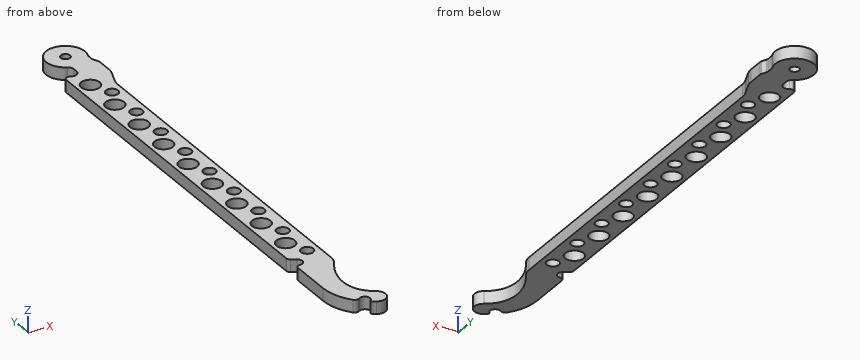
from build123d import *

# Parameters (mm, degrees)
EXTRUDE_1_DEPTH     = 6
CUT_EXTRUDE_1_DEPTH = 7.0000001
HOLE_WIZARD_M41_D   = 4.5
CUT_EXTRUDE_2_DEPTH = 7.0000001
SKETCH_9_R          = 3
SKETCH_9_R_2        = 4.5
CUT_EXTRUDE_4_DEPTH = 7.0000001
CUT_EXTRUDE_6_DEPTH = 7.0000001
FILLET_4_R          = 2
FILLET_5_R          = 10
FILLET_6_R          = 1
FILLET_7_R          = 3


with BuildPart() as part:
    # Эскиз1 → Бобышка-Вытянуть1 (new body)
    with BuildSketch(Plane.XY):
        with BuildLine():
            Line((6.5, -30), (6.5, -210))
            add(Edge.make_bspline(
                [(7.75, -241.602885683), (-4.554007881, -234.499163421), (-0.209884915, -217.844238119), (6.5, -210)],
                knots=[0, 0, 0, 0, 1, 1, 1, 1], degree=3))
            ThreePointArc((7.75, -241.602885683), (9.397114317, -247.75), (3.25, -249.397114317))
            ThreePointArc((3.25, -249.397114317), (1.977735046, -248.713449013), (0.749010369, -247.954310008))
            Line((0.749010369, -247.954310008), (1.25, -247.665063509))
            ThreePointArc((1.25, -247.665063509), (2.165063509, -244.25), (-1.25, -243.334936491))
            Line((-1.25, -243.334936491), (-3.342048726, -244.542781386))
            ThreePointArc((-3.342048726, -244.542781386), (-8.273241088, -236.903089302), (-10, -227.975611669))
            Line((-10, -227.975611669), (-10, 0))
            ThreePointArc((-10, 0), (0, 10), (10, 0))
            Line((10, 0), (10, -20.383829032))
            Line((10, -20.383829032), (6.5, -30))
        make_face()
    extrude(amount=EXTRUDE_1_DEPTH)

    # Эскиз2 → Вырез-Вытянуть1 (cut, through all)
    with BuildSketch(Plane.XY.offset(6)):
        with BuildLine():
            Line((-6.59421021, -201.178331294), (-10, -199.211997642))
            Line((-10, -199.211997642), (-10, -204.985500334))
            Line((-10, -204.985500334), (-9.09421021, -205.508458313))
            ThreePointArc((-9.09421021, -205.508458313), (-5.6791467, -204.593394804), (-6.59421021, -201.178331294))
        make_face()
    extrude(amount=-CUT_EXTRUDE_1_DEPTH, mode=Mode.SUBTRACT)

    # Отверстие с зазором M41 (through all)
    with Locations(Plane.XY.offset(6)):
        with Locations((0, 0)):
            Hole(HOLE_WIZARD_M41_D / 2)

    # Эскиз6 → Вырез-Вытянуть2 (cut, through all)
    with BuildSketch(Plane.XY.offset(6)):
        with BuildLine():
            ThreePointArc((8.758748453, -3.313367558), (-3.216437094, 8.794805936), (-4.554549196, -8.182307784))
            ThreePointArc((-4.554549196, -8.182307784), (-3.004971936, -13.622786652), (-8.445450804, -15.172363912))
            ThreePointArc((-8.445450804, -15.172363912), (-5.964204156, 16.308112544), (16.241251547, -6.143941255))
            ThreePointArc((16.241251547, -6.143941255), (11.084713151, -8.469905953), (8.758748453, -3.313367558))
        make_face()
    extrude(amount=-CUT_EXTRUDE_2_DEPTH, mode=Mode.SUBTRACT)

    # Эскиз9 → Вырез-Вытянуть4 (cut, through all)
    with BuildSketch(Plane.XY.offset(6)):
        with Locations((1, -36.464522083)):
            Circle(SKETCH_9_R)
        with Locations((1, -56.464522083)):
            Circle(SKETCH_9_R)
        with Locations((1, -76.464522083)):
            Circle(SKETCH_9_R)
        with Locations((1, -96.464522083)):
            Circle(SKETCH_9_R)
        with Locations((1, -116.464522083)):
            Circle(SKETCH_9_R)
        with Locations((1, -136.464522083)):
            Circle(SKETCH_9_R)
        with Locations((1, -156.464522083)):
            Circle(SKETCH_9_R)
        with Locations((1, -176.464522083)):
            Circle(SKETCH_9_R)
        with Locations((1, -196.464522083)):
            Circle(SKETCH_9_R)
        with Locations((-3.5, -26.464522083)):
            Circle(SKETCH_9_R_2)
        with Locations((-3.5, -46.464522083)):
            Circle(SKETCH_9_R_2)
        with Locations((-3.5, -66.464522083)):
            Circle(SKETCH_9_R_2)
        with Locations((-3.5, -86.464522083)):
            Circle(SKETCH_9_R_2)
        with Locations((-3.5, -106.464522083)):
            Circle(SKETCH_9_R_2)
        with Locations((-3.5, -126.464522083)):
            Circle(SKETCH_9_R_2)
        with Locations((-3.5, -146.464522083)):
            Circle(SKETCH_9_R_2)
        with Locations((-3.5, -166.464522083)):
            Circle(SKETCH_9_R_2)
        with Locations((-3.5, -186.464522083)):
            Circle(SKETCH_9_R_2)
    extrude(amount=-CUT_EXTRUDE_4_DEPTH, mode=Mode.SUBTRACT)

    # Эскиз11 → Вырез-Вытянуть6 (cut, through all)
    with BuildSketch(Plane.XY.offset(6)):
        Polygon((-2.5, -9.32593934), (-2.5, -18.481802874), (-10, -14.307049262), (-10, -5.151185729), align=None)
        Polygon((10, -7.851153406), (10, -10.804179155), (8.5, -7.681680155), (8.5, -4.728654406), align=None)
    extrude(amount=-CUT_EXTRUDE_6_DEPTH, mode=Mode.SUBTRACT)

    # Скругление4
    fillet_4_edges = [part.edges().sort_by_distance(p)[0] for p in [
        (-3.342048726, -244.542781386, 3),
        (-10, -204.985500334, 3),
        (-10, -199.211997642, 3),
        (8.5, -7.681680155, 3),
        (-10, -14.307049262, 3),
        (10, -10.804179155, 3),
    ]]
    fillet(fillet_4_edges, radius=FILLET_4_R)

    # Скругление5
    fillet_5_edges = [part.edges().sort_by_distance(p)[0] for p in [
        (6.5, -30, 3),
        (6.5, -210, 3),
        (10, -20.383829032, 3),
    ]]
    fillet(fillet_5_edges, radius=FILLET_5_R)

    # Скругление6
    fillet_6_edges = [part.edges().sort_by_distance(p)[0] for p in [
        (0.749010369, -247.954310008, 3),
    ]]
    fillet(fillet_6_edges, radius=FILLET_6_R)

    # Скругление7
    fillet_7_edges = [part.edges().sort_by_distance(p)[0] for p in [
        (-2.5, -9.32593934, 3),
        (-2.5, -18.481802874, 3),
    ]]
    fillet(fillet_7_edges, radius=FILLET_7_R)


solid = part.part
Design review of the part built by this model. Coordinates are the model's own, in mm. Coordinates: 2 decimals unless noted, no trailing zeros. Write each loop counter-clockwise with the first axis right and the second up, starting at its lowest first coordinate (ties: lowest second). Pieces come first, ordered by that corner, then holes. Notation, with made-up numbers: (-26.5, 1) -> (6.5, 1) arc R32 ccw to (6.5, 33) -> close; hole circle Ø5 at (60.5, 36). An arc over 180 degrees is marked (long way). Write each question's results on one line, items separated by ' | '. Start each with the question number.
(1) Take a section at A-A on y = 0. Write out the cut boundary in (x, z), and give its area (3 significant figures).
(2) Clearance check with flat-ended pins moving along their axes: P1, Ø3.5, axis at x = 1, y = -116.46, coming from the -Z side; P2, Ø2, axis at x = 2.5, z = 2.5, coming from the +Y side; P3, Ø3, axis at y = -200, z = 2, coming from the +X side; P4, Ø1.2, axis at y = -5.5, z = 2.5, coming from the +X side. State where each tip first meets the part, or that it passes through.
(3) For line 1 along X through (y, z) = (-147, 4.5); line 2 along X through (y, z) = (-26.5, 4.5); line 3 along X through (y, z) = (-12.5, 4.5), list the stretches that pass through material, from the lowest coordinate up. Write a range as from..to.
(4) Take a section at B-B on z = 4. Give the number of separate pieces and of enclosed holes in the cut face, and give its area (3 significant figures).
Results found:
1) outline: (-9.36, 0) -> (-2.25, 0) -> (-2.25, 6) -> (-9.36, 6) -> close; (2.25, 0) -> (9.36, 0) -> (9.36, 6) -> (2.25, 6) -> close | area: 85.4 mm2
2) P1: passes through | P2: stops at y = 9.24 | P3: stops at x = 6.5 | P4: stops at x = 8.5
3) line 1: x = -10..-7.97, 0.97..6.5 | line 2: x = -10..-8, 1..7.77 | line 3: x = -2.5..10
4) separate pieces: 1 | enclosed holes: 19 | area: 3,170 mm2
